```python
from build123d import *

# Parameters (mm, degrees)
F1_DEPTH = 3.048
F2_R     = 1.1176
F3_DEPTH = 6.35
F4_R     = 5.08


with BuildPart() as f1:
    # F0 (on Top) → F1 (new body, symmetric)
    with BuildSketch(Plane.XY):
        with BuildLine():
            add(Edge.make_bspline(
                [(-25.4, 25.4), (0, 14.75683), (0, 14.75683), (25.4, 25.4)],
                knots=[0, 0, 0, 0, 50.8, 50.8, 50.8, 50.8], degree=3))
            add(Edge.make_bspline(
                [(-25.4, 25.4), (-12.7, -0.009303), (-12.678587, 0), (-25.4, -25.4)],
                knots=[0, 0, 0, 0, 50.8, 50.8, 50.8, 50.8], degree=3))
            Line((-25.4, -25.4), (25.4, -25.4))
            add(Edge.make_bspline(
                [(25.4, 25.4), (12.7, 0), (12.7, 0), (25.4, -25.4)],
                knots=[0, 0, 0, 0, 50.8, 50.8, 50.8, 50.8], degree=3))
        make_face()
    extrude(amount=F1_DEPTH, both=True)

    # F2 (on face) → F3 (cut)
    with BuildSketch(Plane.XY.offset(3.048)):
        with Locations((-17.78, -20.32)):
            Circle(F2_R)
        with Locations((17.78, -20.32)):
            Circle(F2_R)
        with Locations((0, -13.591802)):
            Circle(F2_R)
        with Locations((-10.568528, 0)):
            Circle(F2_R)
        with Locations((10.568528, 0)):
            Circle(F2_R)
    extrude(amount=-F3_DEPTH, mode=Mode.SUBTRACT)

    # F4
    f4_edges = [f1.edges().sort_by_distance(p)[0] for p in [
        (-25.4, -25.4, -1.524),
        (25.4, -25.4, -1.524),
    ]]
    fillet(f4_edges, radius=F4_R)


solid = f1.part
```
Geometry check sheet. Reference: the model listing, model coordinates, mm. Give positions to 0.01 mm unless a question says otherwise; leave off trailing zeros. Write each question's results on one line, items separated by ' | '. Start each with the question number.
(1) Sectioned sample at A-A (y = -20.32). Give the number of separate pieces and of enclosed holes in the cut face, plus the area to 3 significant figures.
(2) Gauge pin test, flat ends, axial feed: P1, Ø1, axis at x = -11.5, z = -0.5, coming from the +Y side; P2, Ø1, axis at y = -5.5, z = 0.5, coming from the -X side. Record the tip position at first contact, or that the pin passes through.
(3) Mould release check, pull along X, two halves, no side actions. Record for faces 1 (the face through (18.381, -19.378, 0.043)), 2 (the face through (0, 0, 3.048)): pulls with the +X half, pulls with the -X half, needs draft (parallel to the pull), parting line crosses it, or undercut.
(4) Scan lines: line 1 (Y direction, x = 0, z = 0.25); line 2 (X direction, y = -20, z = 2.5); line 3 (Y direction, x = 20, z = 1.5). Record each from-to range of solid material in increasing order.
Answer below:
1) separate pieces: 3 | enclosed holes: 0 | area: 244 mm2
2) P1: y = 20 | P2: x = -16.75
3) face 1: undercut | face 2: needs draft
4) line 1: -25.4 to -14.71, -12.47 to 17.42 | line 2: -22.28 to -18.85, -16.71 to 16.71, 18.85 to 22.28 | line 3: -24.57 to -14.35, 14.35 to 23.15
